Could you check a few things on this drawing? It's one solid part, dimensions in mm from its lowest x, y, z. A direction names the side the tool comes from. Give positions to 0.01 mm unless a question says otherwise; leave off trailing zeros. Loops run counter-clockwise (first coordinate to the right, second up) from the corner with the lowest first, then second, coordinate; pieces in that order, holes last. Notation, with made-up numbers: (-36, -36.5) - (20, -36.5) arc R30 ccw to (20, 1.5) - close; hole circle Ø6 at (83, 14.25). An arc over 180 degrees is marked (long way). Return JSON: item names as keys, results as strings. Group by question number.
(1) I need wall thicknesses on probe 1 along Z at (x, y) = (4.25, 0.5); probe 2 along X at (y, z) = (3, 11.75); probe 3 along X at (y, z) = (3, 23.5). Which ranges of each line are inside material? Lowest first, please. Write a range as [from, to].
(2) For P1, Ø3, axis at y = 2, z = 5, coming from the +X side; P2, Ø1.5, axis at y = 5, z = 11.5, coming from the +X side (1 decimal); P3, Ø1.5, axis at x = 1.5, z = 18.5, coming from the +Y side, each with a flat end and sliding along its axis, tell me the tip position at first contact or that it passes through.
(3) If we section it at A-A (x = 5): Please give me the cut outline in (y, z).
(4) On a 3-axis mill with a long thin cutter (end or side, diameter ignored), from which of +Z, -Z, +X, -X, +Y, -Y can I reach the whole of each face in a straight line? I mean the marked faces 1 and 2. Say none if no direction works.
(5) If we section it at C-C (z = 10.75): Please give me the cut outline in (x, y) (1 decimal), then the cut area to 3 significant figures.
(6) If we section it at D-D (z = 21): Please give me the cut outline in (x, y) (1 decimal).
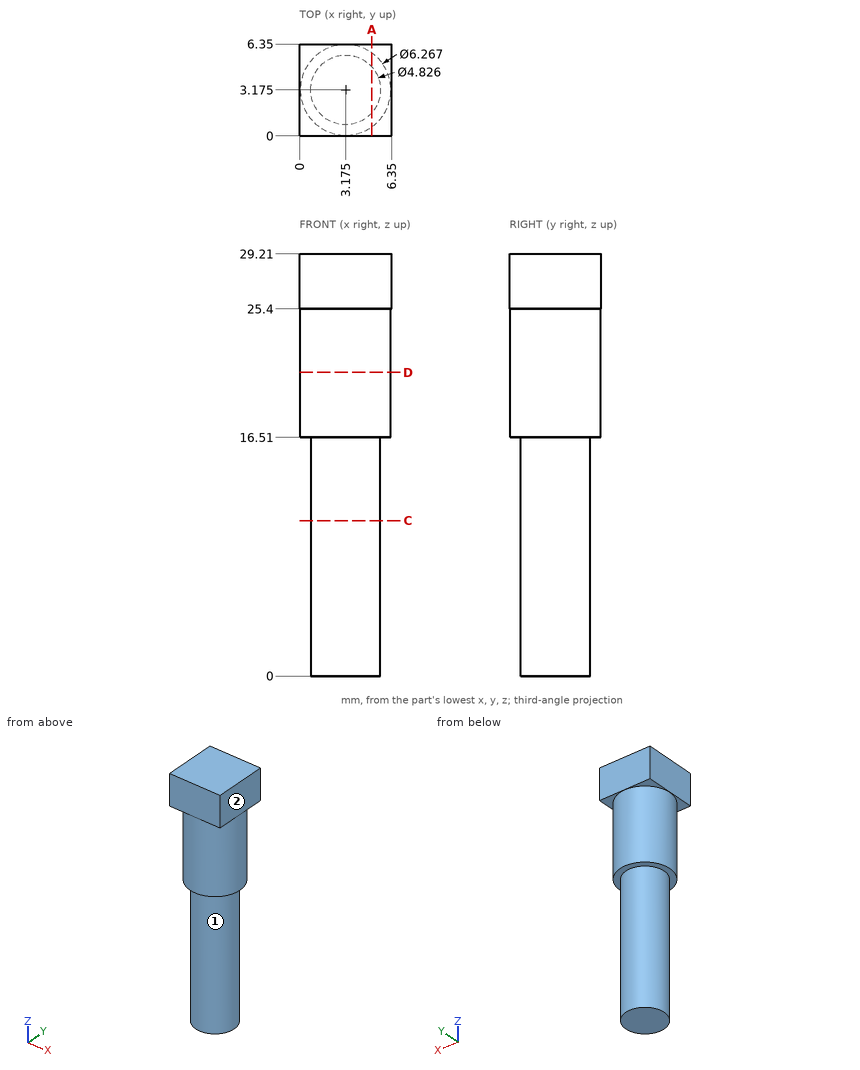
Values:
{
 "1": {"probe 1": "[16.51, 29.21]", "probe 2": "[0.77, 5.58]", "probe 3": "[0.05, 6.3]"},
 "2": {"P1": "x = 5.59", "P2": "x = 5.3", "P3": "y = 6.17"},
 "3": {"outline": "(0, 25.4) - (0.63, 25.4) - (0.63, 16.51) - (1.6, 16.51) - (1.6, 0) - (4.75, 0) - (4.75, 16.51) - (5.72, 16.51) - (5.72, 25.4) - (6.35, 25.4) - (6.35, 29.21) - (0, 29.21) - close"},
 "4": {"face 1": "-Z", "face 2": "+Z, -Z, +X, +Y, -Y"},
 "5": {"outline": "circle Ø4.8 at (3.2, 3.2)", "area": "18.3 mm2"},
 "6": {"outline": "circle Ø6.3 at (3.2, 3.2)"}
}
